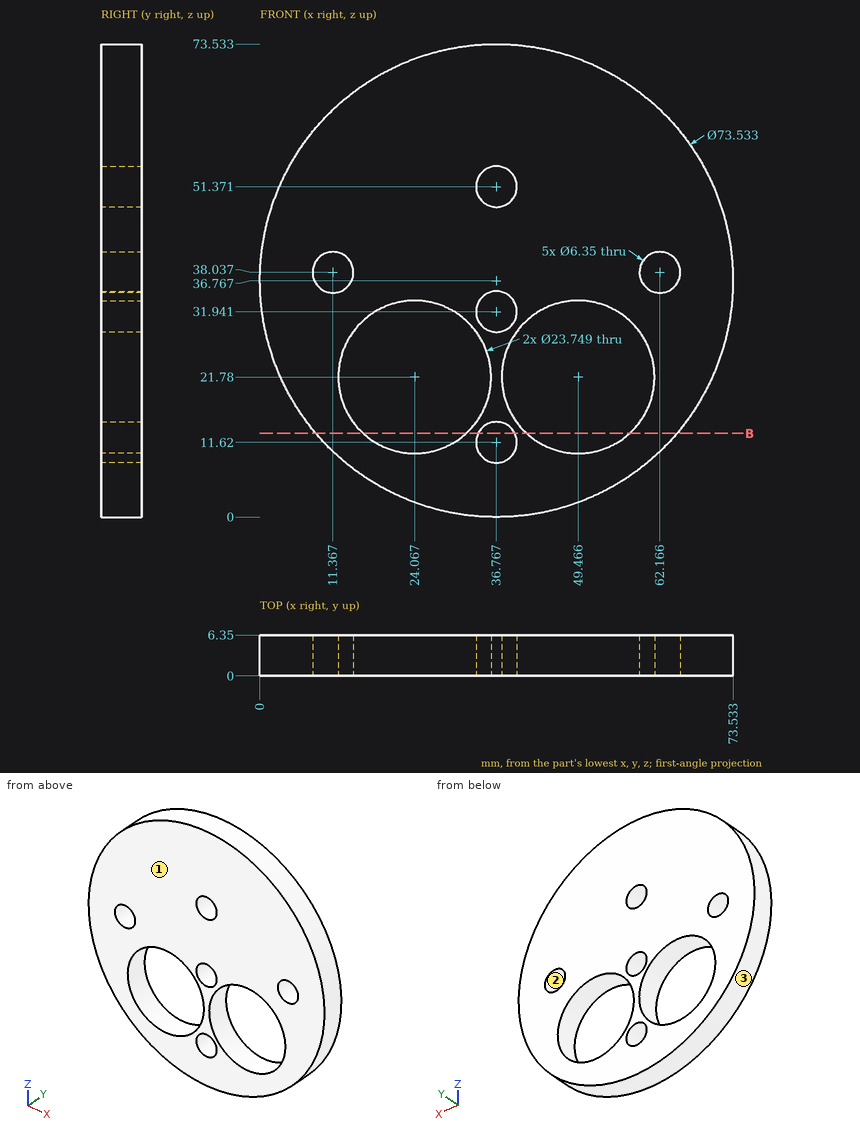
For this review, use the dimensioned drawing (mm, ordinates from the lowest corner) and the shaded views. Coordinates: 2 decimals unless noted, no trailing zeros. Use one line per item in the form item = value.
Q1. Draft analysis for pull direction Z (two halves, no side actions). For the marked faces 1, 2 and 3, state which applies: +Z half, -Z half, draft (parallel to the pull), parting line (faces both ways), or undercut.
Checked values:
face_1 = draft
face_2 = undercut
face_3 = parting line
Q2. For P1, Ø4, axis at x = 65, z = 12, coming from the +Y side; P2, Ø4, axis at x = 36.77, z = 31.94, coming from the -Y side; P3, Ø2, axis at x = 9, y = 5.5, coming from the +Z side; P4, Ø1.5, axis at x = 44.5, y = 3.5, coming from the +Z side, all flat-tipped, find the tip position at first contact; note any pin that passes through.
Checked values:
P1 = 6.35
P2 = through
P3 = 61.97
P4 = 72.86
Q3. For probe 1 along X at (y, z) = (2.5, 28); probe 2 along X at (y, z) = (4, 17) (1 decimal); probe 3 along Z at (x, y) = (44, 2.5) (1 decimal), list the stretches that pass through material, from the lowest coordinate up. Write a range as from..to.
Checked values:
probe_1 = 1.06..13.95, 34.18..39.35, 59.58..72.47
probe_2 = 5.8..13.2, 34.9..38.6, 60.3..67.8
probe_3 = 0.7..11.2, 32.3..72.8
Q4. Consider section B-B (z = 13). Give the number of separate pieces and of enclosed holes in the cut face, then the cut area to 3 significant figures.
Checked values:
separate_pieces = 4
enclosed_holes = 0
area = 117 mm2
